```python
from build123d import *

# Parameters (mm, degrees)
SKETCH1_W             = 58.166
SKETCH1_H             = 28.448
BOSS_EXTRUDE1_DEPTH   = 21.844
SKETCH2_W             = 55.626
SKETCH2_H             = 24.638
CUT_EXTRUDE1_DEPTH    = 40.055132838
SKETCH3_W             = 3.048
SKETCH3_H             = 2.413
SKETCH3_W_2           = 10.668
BOSS_EXTRUDE2_DEPTH   = 0.762
F_2_CLEARANCE_HOLE1_D = 2.7051
CUT_EXTRUDE2_REACH    = 48.177
SKETCH6_W             = 10.16
SKETCH6_H             = 2.54
SKETCH7_W             = 58.166
SKETCH7_H             = 21.844
BOSS_EXTRUDE3_DEPTH   = 3.81
CUT_EXTRUDE3_REACH    = 50.616
SKETCH8_W             = 53.086
SKETCH8_H             = 10.16


with BuildPart() as part:
    # Sketch1 → Boss-Extrude1 (new body)
    with BuildSketch(Plane(origin=(0, 0, 0), x_dir=(1, 0, 0), z_dir=(0, 1, 0))):
        Rectangle(SKETCH1_W, SKETCH1_H)
    extrude(amount=BOSS_EXTRUDE1_DEPTH)

    # Sketch2 → Cut-Extrude1 (cut, through all)
    with BuildSketch(Plane(origin=(0, 21.844, 0), x_dir=(1, 0, 0), z_dir=(0, 1, 0))):
        Rectangle(SKETCH2_W, SKETCH2_H)
    extrude(amount=-CUT_EXTRUDE1_DEPTH, mode=Mode.SUBTRACT)

    # Sketch3 → Boss-Extrude2 (add)
    with BuildSketch(Plane(origin=(0, 21.844, 0), x_dir=(1, 0, 0), z_dir=(0, 1, 0))):
        with Locations((-26.289, 11.1125)):
            Rectangle(SKETCH3_W, SKETCH3_H)
        with Locations((-26.289, -11.1125)):
            Rectangle(SKETCH3_W, SKETCH3_H)
        with Locations((26.289, 11.1125)):
            Rectangle(SKETCH3_W, SKETCH3_H)
        with Locations((26.289, -11.1125)):
            Rectangle(SKETCH3_W, SKETCH3_H)
        with Locations((-0.127, 11.1125)):
            Rectangle(SKETCH3_W_2, SKETCH3_H)
        with Locations((-0.127, -11.1125)):
            Rectangle(SKETCH3_W_2, SKETCH3_H)
    extrude(amount=-BOSS_EXTRUDE2_DEPTH)

    # #2 Clearance Hole1 (through all)
    with Locations(Plane(origin=(0, 21.844, 0), x_dir=(1, 0, 0), z_dir=(0, 1, 0))):
        with Locations((-27.051, 12.0015), (-3.05054, 12.0015), (-3.05054, -11.99896), (-27.051, -11.99896), (2.91846, -11.99896), (26.91892, -11.99896), (26.91892, 12.0015), (2.91846, 12.0015)):
            Hole(F_2_CLEARANCE_HOLE1_D / 2)

    # Sketch6 → Cut-Extrude2 (cut, up to next)
    with BuildSketch(Plane.XY.offset(14.224), mode=Mode.PRIVATE) as cut_extrude2_sk1:
        with Locations((-13.843, 1.27)):
            Rectangle(SKETCH6_W, SKETCH6_H)
    cut_extrude2_tool1 = extrude(cut_extrude2_sk1.sketch, amount=-CUT_EXTRUDE2_REACH, mode=Mode.PRIVATE) & part.part
    # Sketch6 → Cut-Extrude2 (cut, up to next)
    with BuildSketch(Plane.XY.offset(14.224), mode=Mode.PRIVATE) as cut_extrude2_sk2:
        with Locations((12.827, 1.27)):
            Rectangle(SKETCH6_W, SKETCH6_H)
    cut_extrude2_tool2 = extrude(cut_extrude2_sk2.sketch, amount=-CUT_EXTRUDE2_REACH, mode=Mode.PRIVATE) & part.part
    add(cut_extrude2_tool1.solids().sort_by_distance((-13.843, 1.27, 14.224))[0], mode=Mode.SUBTRACT)
    add(cut_extrude2_tool2.solids().sort_by_distance((12.827, 1.27, 14.224))[0], mode=Mode.SUBTRACT)

    # Sketch7 → Boss-Extrude3 (add)
    with BuildSketch(Plane(origin=(0, 0, -14.224), x_dir=(-1, 0, 0), z_dir=(0, 0, -1))):
        with Locations((0, 10.922)):
            Rectangle(SKETCH7_W, SKETCH7_H)
    extrude(amount=BOSS_EXTRUDE3_DEPTH)

    # Sketch8 → Cut-Extrude3 (cut, up to next)
    with BuildSketch(Plane(origin=(0, 0, -18.034), x_dir=(-1, 0, 0), z_dir=(0, 0, -1)), mode=Mode.PRIVATE) as cut_extrude3_sk1:
        with Locations((0, 5.08)):
            Rectangle(SKETCH8_W, SKETCH8_H)
    cut_extrude3_tool1 = extrude(cut_extrude3_sk1.sketch, amount=-CUT_EXTRUDE3_REACH, mode=Mode.PRIVATE) & part.part
    add(cut_extrude3_tool1.solids().sort_by_distance((0, 5.08, -18.034))[0], mode=Mode.SUBTRACT)


solid = part.part
```
For this review, take the finished solid that the model builds, in its own axes (mm). A direction names the side the tool comes from. Give positions to 0.01 mm unless a question says otherwise; leave off trailing zeros. Order: outer loops, then holes, each group sorted by start corner. A loop starts at its lowest first (then second) coordinate and runs counter-clockwise, first axis right, second up.
1) Take a section at C-C (z = 7). Give the boundary of the cut face in (x, y).
2) Take a section at D-D (y = 3.25). Give the boundary of the cut face in (x, z).
3) Insertion check: pin 1 (1 mm diameter, centred on x = 11.5, z = 13.5, fed in from -Y); pin 2 (3 mm diameter, centred on x = -1.5, z = -15.5, fed in from -Y); pin 3 (1.2 mm diameter, centred on x = -25.5, z = 10.5, fed in from -Y). Each pin has a flat end and moves straight along its axis. Give the tip position at first contact, or say it passes through.
4) The part is to be moulded in two halves that separate along Z. For faces 1 (the face through (0, 21.082, -11)), 2 (the face through (-2, 21.844, -10.2)), say which applies: released by +Z, released by -Z, zero draft, split by the parting line, or undercut.
5) Take a section at A-A (x = 11). Give the boundary of the cut face in (y, z), then the cut area to 3 significant figures.
6) Wall thickness on line 1 (Z direction, x = -21.5, y = 17); line 2 (X direction, y = 3.75, z = 2); line 3 (X direction, y = 11.5, z = 12): over which ranges is each line inside the solid? List them lowest first.
7) Take a section at B-B (y = 13.75). Give the boundary of the cut face in (x, z).
8) For faces 3 (the face through (-26.543, 5, -16)), 4 (the face through (7.747, 1, 13)), 5 (the face through (25.9, 21.082, 10.8)), 6 (the face through (27.916, 10.769, -12.916)), list the 3-axis set-ups (+Z, -Z, +X, -X, +Y, -Y) from which the entire face can be reached by the end or side of a thin tool; tool diameter is ignored.
Derived:
1. outline: (-29.08, 0) - (-27.81, 0) - (-27.81, 21.84) - (-29.08, 21.84) - close; (27.81, 0) - (29.08, 0) - (29.08, 21.84) - (27.81, 21.84) - close
2. outline: (-29.08, -18.03) - (-26.54, -18.03) - (-26.54, -13.26) arc R1.35 cw to (-27.81, -10.88) - (-27.81, 10.88) arc R1.35 cw (long way) to (-25.74, 12.32) - (-4.36, 12.32) arc R1.35 cw to (-1.74, 12.32) - (1.6, 12.32) arc R1.35 cw to (4.23, 12.32) - (25.6, 12.32) arc R1.35 cw (long way) to (27.81, 10.98) - (27.81, -10.99) arc R1.35 cw to (26.54, -13.3) - (26.54, -18.03) - (29.08, -18.03) - (29.08, 14.22) - (-29.08, 14.22) - close
3. pin 1: stops at y = 2.54
3. pin 2: stops at y = 10.16
3. pin 3: stops at y = 21.08
4. face 1: undercut
4. face 2: zero draft
5. outline: (2.54, 12.32) - (21.84, 12.32) - (21.84, 14.22) - (2.54, 14.22) - close; (10.16, -18.03) - (21.84, -18.03) - (21.84, -12.32) - (10.16, -12.32) - close
5. area: 104 mm2
6. line 1: z = -18.03 to -12.32, 12.32 to 14.22
6. line 2: x = -29.08 to -27.81, 27.81 to 29.08
6. line 3: x = -29.08 to -28.4, 28.27 to 29.08
7. outline: (-29.08, -18.03) - (29.08, -18.03) - (29.08, 14.22) - (-29.08, 14.22) - close; hole (-27.81, -10.88) arc R1.35 ccw (long way) to (-25.74, -12.32) - (-4.37, -12.32) arc R1.35 ccw to (-1.74, -12.32) - (1.6, -12.32) arc R1.35 ccw to (4.23, -12.32) - (25.6, -12.32) arc R1.35 ccw (long way) to (27.81, -10.99) - (27.81, 10.98) arc R1.35 ccw (long way) to (25.6, 12.32) - (4.23, 12.32) arc R1.35 ccw to (1.6, 12.32) - (-1.74, 12.32) arc R1.35 ccw to (-4.36, 12.32) - (-25.74, 12.32) arc R1.35 ccw (long way) to (-27.81, 10.88) - close
8. face 3: -Z, -Y
8. face 4: +Z, -Z, -Y
8. face 5: -Y
8. face 6: +Y, -Y
